CAD build for the part. Positions are in the model's coordinates, mm. A direction names the side the tool comes from. Give positions to 0.01 mm unless a question says otherwise; leave off trailing zeros. Write each loop counter-clockwise with the first axis right and the second up, starting at its lowest first coordinate (ties: lowest second). Pieces come first, ordered by that corner, then holes. Notation, with made-up numbers: (39.5, 10.5) -> (88.5, 10.5) arc R12 ccw to (88.5, 18.5) -> close; hole circle Ø2 at (45, 50.25). An arc over 180 degrees is marked (long way). Use one line per item in the form item = value. Start each with the question number.
from build123d import *

# Parameters (mm, degrees)
SKETCH1_R           = 3.6
SKETCH1_R_2         = 2.5
SKETCH1_R_3         = 1.5
BOSS_EXTRUDE1_DEPTH = 1.25
SKETCH2_R           = 2
SKETCH2_R_2         = 1.5
BOSS_EXTRUDE2_DEPTH = 1.5
SKETCH3_R           = 2.7
SKETCH3_R_2         = 1.5
BOSS_EXTRUDE3_DEPTH = 4.5
FILLET1_R           = 10
SKETCH4_W           = 17
SKETCH4_H           = 2.5
BOSS_EXTRUDE4_DEPTH = 22.9
SKETCH5_W           = 1.5
SKETCH5_H           = 11
CUT_EXTRUDE1_DEPTH  = 20.1
FILLET2_R           = 2


with BuildPart() as part:
    # Sketch1 → Boss-Extrude1 (new body, symmetric)
    with BuildSketch(Plane.XY):
        with BuildLine():
            Line((-12, -28.35), (-12, -23.75))
            Line((-12, -23.75), (-32, -23.75))
            Line((-32, -23.75), (-32, 23.75))
            Line((-32, 23.75), (32, 23.75))
            Line((32, 23.75), (32, -23.75))
            Line((32, -23.75), (12, -23.75))
            Line((12, -23.75), (12, -28.35))
            ThreePointArc((12, -28.35), (0, -40.35), (-12, -28.35))
        make_face()
        with Locations((0, -28.35)):
            Circle(SKETCH1_R, mode=Mode.SUBTRACT)
        with Locations((-20, 11.85)):
            Circle(SKETCH1_R_2, mode=Mode.SUBTRACT)
        with Locations((19, -9.5)):
            Circle(SKETCH1_R_3, mode=Mode.SUBTRACT)
        with Locations((1.5, 9.4)):
            Circle(SKETCH1_R_3, mode=Mode.SUBTRACT)
        with Locations((20, 11.85)):
            Circle(SKETCH1_R_2, mode=Mode.SUBTRACT)
        with Locations((-23.5, -0.7)):
            Circle(SKETCH1_R_3, mode=Mode.SUBTRACT)
        with Locations((-9.5, -0.7)):
            Circle(SKETCH1_R_3, mode=Mode.SUBTRACT)
    extrude(amount=BOSS_EXTRUDE1_DEPTH, both=True)

    # Sketch2 → Boss-Extrude2 (add)
    with BuildSketch(Plane.XY.offset(1.25)):
        with Locations((19, -9.5)):
            Circle(SKETCH2_R)
        with Locations((19, -9.5)):
            Circle(SKETCH2_R_2, mode=Mode.SUBTRACT)
        with Locations((1.5, 9.4)):
            Circle(SKETCH2_R)
        with Locations((1.5, 9.4)):
            Circle(SKETCH2_R_2, mode=Mode.SUBTRACT)
    extrude(amount=BOSS_EXTRUDE2_DEPTH)

    # Sketch3 → Boss-Extrude3 (add)
    with BuildSketch(Plane(origin=(0, 0, -1.25), x_dir=(-1, 0, 0), z_dir=(0, 0, -1))):
        with Locations((9.5, -0.7)):
            Circle(SKETCH3_R)
        with Locations((9.5, -0.7)):
            Circle(SKETCH3_R_2, mode=Mode.SUBTRACT)
        with Locations((23.5, -0.7)):
            Circle(SKETCH3_R)
        with Locations((23.5, -0.7)):
            Circle(SKETCH3_R_2, mode=Mode.SUBTRACT)
    extrude(amount=BOSS_EXTRUDE3_DEPTH)

    # Fillet1
    fillet1_edges = [part.edges().sort_by_distance(p)[0] for p in [
        (-32, 23.75, 0),
        (32, 23.75, 0),
    ]]
    fillet(fillet1_edges, radius=FILLET1_R)

    # Sketch4 → Boss-Extrude4 (add)
    with BuildSketch(Plane.XY.offset(1.25)):
        with Locations((-23.5, -22.5)):
            Rectangle(SKETCH4_W, SKETCH4_H)
        with Locations((23.5, -22.5)):
            Rectangle(SKETCH4_W, SKETCH4_H)
    extrude(amount=BOSS_EXTRUDE4_DEPTH)

    # Sketch5 → Cut-Extrude1 (cut, through all)
    with BuildSketch(Plane(origin=(0, -21.25, 0), x_dir=(1, 0, 0), z_dir=(0, 1, 0))):
        with Locations((-20.75, -18.65)):
            Rectangle(SKETCH5_W, SKETCH5_H)
        with Locations((20.75, -18.65)):
            Rectangle(SKETCH5_W, SKETCH5_H)
    extrude(amount=-CUT_EXTRUDE1_DEPTH, mode=Mode.SUBTRACT)

    # Fillet2
    fillet2_edges = [part.edges().sort_by_distance(p)[0] for p in [
        (32, -22.5, 24.15),
        (15, -22.5, 24.15),
        (-32, -22.5, 24.15),
        (-15, -22.5, 24.15),
    ]]
    fillet(fillet2_edges, radius=FILLET2_R)


solid = part.part
1) Two-plate mould, pull along Y, no slides. Class faces 5 (the face through (1.305, 10.887, 0.722)), 6 (the face through (-11, -2, -5.75)), 7 (the face through (-22, -23.75, 11)): released by +Y, released by -Y, zero draft, split by the parting line, or undercut.
2) Wall check: line 1 along X through (y, z) = (-0.7, 0.1); line 2 along Y through (x, z) = (-9.5, -2.6); line 3 along Y through (x, z) = (19, 1.55). Give the ranges that are in metal, low to high. Write a range as from..to.
3) Cut at C-C (z = 5.75). Give the cut face in (x, y).
4) Cut at A-A (z = 14). Give the cut face in (x, y).
5) Cut at B-B (y = -9.5). Give the cut face in (x, z).
6) Cut at D-D (x = 1.5). Give the cut face in (y, z).
7) 3-axis set-ups, long thin cutter, end or side, ignore diameter. For faces 1 (the face through (20, -8, 2.75)), 2 (the face through (21, -22, 13.15)), 3 (the face through (2.423, 7.626, 1.99)), 4 (the face through (-12.075, 0.111, -3.468)): which of +Z, -Z, +X, -X, +Y, -Y reach the whole face in a straight line?
8) Pin check, flat tips, straight feed: pin 1 (1 mm diameter, centred on y = -3, z = -2, fed in from -X); pin 2 (5 mm diameter, centred on x = 1.5, y = 9.4, fed in from -Z); pin 3 (4 mm diameter, centred on x = 12.5, y = 15, fed in from +Z). Stop position of each tip, or through.
Final values:
q1.face_5 = undercut
q1.face_6 = zero draft
q1.face_7 = released by -Y
q2.line_1 = -32..-25, -22..-11, -8..32
q2.line_2 = -3.4..-2.2, 0.8..2
q2.line_3 = -23.75..-21.25, -11.5..-11, -8..-7.5
q3.outline = (-32, -23.75) -> (-15, -23.75) -> (-15, -21.25) -> (-32, -21.25) -> close; (15, -23.75) -> (32, -23.75) -> (32, -21.25) -> (15, -21.25) -> close
q4.outline = (-32, -23.75) -> (-21.5, -23.75) -> (-21.5, -21.25) -> (-32, -21.25) -> close; (-20, -23.75) -> (-15, -23.75) -> (-15, -21.25) -> (-20, -21.25) -> close; (15, -23.75) -> (20, -23.75) -> (20, -21.25) -> (15, -21.25) -> close; (21.5, -23.75) -> (32, -23.75) -> (32, -21.25) -> (21.5, -21.25) -> close
q5.outline = (-32, -1.25) -> (17.5, -1.25) -> (17.5, 2.75) -> (17, 2.75) -> (17, 1.25) -> (-32, 1.25) -> close; (20.5, -1.25) -> (32, -1.25) -> (32, 1.25) -> (21, 1.25) -> (21, 2.75) -> (20.5, 2.75) -> close
q6.outline = (-40.26, -1.25) -> (-31.62, -1.25) -> (-31.62, 1.25) -> (-40.26, 1.25) -> close; (-25.08, -1.25) -> (7.9, -1.25) -> (7.9, 2.75) -> (7.4, 2.75) -> (7.4, 1.25) -> (-25.08, 1.25) -> close; (10.9, -1.25) -> (23.75, -1.25) -> (23.75, 1.25) -> (11.4, 1.25) -> (11.4, 2.75) -> (10.9, 2.75) -> close
q7.face_1 = +Z, +X, -X, +Y
q7.face_2 = +Z, +Y, -Y
q7.face_3 = +Z
q7.face_4 = -Z
q8.pin_1 = -25.51
q8.pin_2 = -1.25
q8.pin_3 = 1.25
